Geometry: final body of the model. Coordinates: model frame, mm. A direction names the side the tool comes from. Give positions to 0.01 mm unless a question says otherwise; leave off trailing zeros. Write each loop counter-clockwise with the first axis right and the second up, starting at its lowest first coordinate (ties: lowest second). Pieces come first, ordered by that corner, then holes.
Q1. Cut plane C-C on x = 56. Return the cut outline in (y, z), plus the area to 3 significant figures.
Q2. Draft query along X for faces 1 (the face through (48.505, 27.242, 9.916)), 2 (the face through (-59.495, -26.758, 9.916)), 3 (the face through (-68, 0, 10)), 4 (the face through (68, 0, 10)). Return one class per face: pulls with the +X half, pulls with the -X half, needs draft (parallel to the pull), parting line crosses it, or undercut.
Q3. Reachability of faces 5 (the face through (30, -1, 2)), 6 (the face through (-30, -1, 2)), 7 (the face through (0, -1, 12)), 8 (the face through (64, 39.8, 10.1)), 9 (the face through (-59.495, 27.242, 9.916)) from +Z, -Z, +X, -X, +Y, -Y: full face, straight path, thin tool, end or side. Return the list, or none.
Q4. Cut plane A-A on y = 27. Return the cut outline in (x, z), plus the area to 3 significant figures.
Q5. Line query: L1, parallel to X at y = 27, z = 10; L2, parallel to Y at x = -54, z = 7.25; L3, parallel to X at y = 22.5, z = 10.75. Output: solid intervals per line, ascending.
Q6. Pin query (flat end, axial travel): pin 1 (11.5 mm diameter, centred on x = -40, y = 8.5, fed in from -Z); pin 2 (4.5 mm diameter, centred on y = -4, z = 1.5, fed in from +X); pin 3 (6 mm diameter, centred on x = -17, y = 27.5, fed in from +Z). Return the tip coordinate at first contact, or that it passes through.
Q7. Cut plane D-D on y = -5.5. Return the cut outline in (x, z), plus the area to 3 significant figures.
Q8. Cut plane B-B on z = 6.75. Return the cut outline in (x, y), plus the area to 3 significant figures.
```python
from build123d import *

# Parameters (mm, degrees)
F1_DEPTH = 44
F2_R     = 14
F3_R     = 5.5
F4_DEPTH = 16.001


with BuildPart() as f1:
    # F0 (on Front) → F1 (new body, symmetric)
    with BuildSketch(Plane.XZ):
        with BuildLine():
            Line((-30, 4), (-30, 0))
            Line((-30, 0), (30, 0))
            Line((30, 0), (30, 4))
            Line((30, 4), (68, 4))
            Line((68, 4), (68, 16))
            Line((68, 16), (24, 16))
            Line((24, 16), (24, 15))
            ThreePointArc((24, 15), (23.12132, 12.87868), (21, 12))
            Line((21, 12), (-21, 12))
            ThreePointArc((-21, 12), (-23.12132, 12.87868), (-24, 15))
            Line((-24, 15), (-24, 16))
            Line((-24, 16), (-68, 16))
            Line((-68, 16), (-68, 4))
            Line((-68, 4), (-30, 4))
        make_face()
    extrude(amount=F1_DEPTH, both=True)

    # F2
    f2_edges = [f1.edges().sort_by_distance(p)[0] for p in [
        (-68, -44, 10),
        (-68, 44, 10),
        (68, 44, 10),
        (68, -44, 10),
    ]]
    fillet(f2_edges, radius=F2_R)

    # F3 (on Top) → F4 (cut, through all)
    with BuildSketch(Plane.XY):
        with Locations((-54, 27)):
            Circle(F3_R)
        with Locations((-54, -27)):
            Circle(F3_R)
        with Locations((54, 27)):
            Circle(F3_R)
        with Locations((54, -27)):
            Circle(F3_R)
    extrude(amount=F4_DEPTH, mode=Mode.SUBTRACT)


solid = f1.part
```
Data:
1. outline: (-43.86, 4) - (-32.12, 4) - (-32.12, 16) - (-43.86, 16) - close; (-21.88, 4) - (21.88, 4) - (21.88, 16) - (-21.88, 16) - close; (32.12, 4) - (43.86, 4) - (43.86, 16) - (32.12, 16) - close
1. area: 807 mm2
2. face 1: undercut
2. face 2: undercut
2. face 3: pulls with the -X half
2. face 4: pulls with the +X half
3. face 5: -Z, +X, +Y, -Y
3. face 6: -Z, -X, +Y, -Y
3. face 7: +Z, +Y, -Y
3. face 8: +Z, -Z, +X, +Y
3. face 9: +Z, -Z
4. outline: (-68, 4) - (-59.5, 4) - (-59.5, 16) - (-68, 16) - close; (-48.5, 4) - (-30, 4) - (-30, 0) - (30, 0) - (30, 4) - (48.5, 4) - (48.5, 16) - (24, 16) - (24, 15) arc R3 cw to (21, 12) - (-21, 12) arc R3 cw to (-24, 15) - (-24, 16) - (-48.5, 16) - close; (59.5, 4) - (68, 4) - (68, 16) - (59.5, 16) - close
4. area: 1,420 mm2
5. L1: x = -68 to -59.5, -48.5 to 48.5, 59.5 to 68
5. L2: y = -44 to -32.5, -21.5 to 21.5, 32.5 to 44
5. L3: x = -68 to -57.16, -50.84 to 50.84, 57.16 to 68
6. pin 1: stops at z = 4
6. pin 2: stops at x = 30
6. pin 3: stops at z = 12
7. outline: (-68, 4) - (-30, 4) - (-30, 0) - (30, 0) - (30, 4) - (68, 4) - (68, 16) - (24, 16) - (24, 15) arc R3 cw to (21, 12) - (-21, 12) arc R3 cw to (-24, 15) - (-24, 16) - (-68, 16) - close
7. area: 1,680 mm2
8. outline: (-68, -30) arc R14 ccw to (-54, -44) - (54, -44) arc R14 ccw to (68, -30) - (68, 30) arc R14 ccw to (54, 44) - (-54, 44) arc R14 ccw to (-68, 30) - close; hole circle Ø11 at (-54, -27); hole circle Ø11 at (-54, 27); hole circle Ø11 at (54, -27); hole circle Ø11 at (54, 27)
8. area: 11,400 mm2
